from build123d import *

# Parameters (mm, degrees)
CYLINDER031_R              = 3.1
CYLINDER031_DEPTH          = 32.5
EXTRUDE002_DEPTH           = 10
CYLINDER038_R              = 2.5
CYLINDER038_DEPTH          = 23
CYLINDER032_R              = 4
CYLINDER032_DEPTH          = 10
EXTRUDE005_DEPTH           = 4
EXTRUDE005_PLACEMENT_ANGLE = 90
CYLINDER019_R              = 11.1
CYLINDER019_DEPTH          = 10
CYLINDER015_R              = 1.6
CYLINDER015_DEPTH          = 10
CYLINDER016_R              = 1.6
CYLINDER016_DEPTH          = 10
CYLINDER017_R              = 1.6
CYLINDER017_DEPTH          = 10
CYLINDER018_R              = 1.6
CYLINDER018_DEPTH          = 10
BOX002_W                   = 44
BOX002_H                   = 4
BOX002_DEPTH               = 43
EXTRUDE001_DEPTH           = 4
EXTRUDE006_DEPTH           = 5.9
EXTRUDE006_PLACEMENT_ANGLE = 90
CYLINDER021_R              = 6
CYLINDER021_DEPTH          = 6
CYLINDER020_R              = 2.1
CYLINDER020_DEPTH          = 10
BOX003_W                   = 66
BOX003_H                   = 25
BOX003_DEPTH               = 4
BOX_W                      = 19
BOX_H                      = 25
BOX_DEPTH                  = 4
CYLINDER028_R              = 11.1
CYLINDER028_DEPTH          = 10
CYLINDER025_R              = 1.6
CYLINDER025_DEPTH          = 10
CYLINDER024_R              = 1.6
CYLINDER024_DEPTH          = 10
CYLINDER023_R              = 1.6
CYLINDER023_DEPTH          = 10
CYLINDER029_R              = 1.6
CYLINDER029_DEPTH          = 10
BOX005_W                   = 44
BOX005_H                   = 4
BOX005_DEPTH               = 43


with BuildPart() as cylinder031:
    # Cylinder031 → Cylinder031 (new body)
    with BuildSketch(Plane(origin=(7.1, -2.84478, 23.5), x_dir=(1, 0, 0), z_dir=(0, 1, 0))):
        Circle(CYLINDER031_R)
    extrude(amount=CYLINDER031_DEPTH)


with BuildPart() as extrude002:
    # Sketch001 → Extrude002 (new body)
    with BuildSketch(Plane.XY):
        with BuildLine():
            ThreePointArc((35.736492, 10), (36.2, 15), (35.736492, 20))
            ThreePointArc((35.736492, 20), (33.490746, 22.111711), (31.244999, 20))
            ThreePointArc((31.244999, 10), (31.8, 15), (31.244999, 20))
            ThreePointArc((31.244999, 10), (33.490746, 7.888289), (35.736492, 10))
        make_face()
    extrude(amount=-EXTRUDE002_DEPTH)


with BuildPart() as extrude002_1:
    # Extrude002 placement: moved
    add(extrude002.part.moved(Location((0, 0, 8))))


with BuildPart() as cylinder038:
    # Cylinder038 → Cylinder038 (new body)
    with BuildSketch(Plane(origin=(6, 27, 39), x_dir=(1, 0, 0), z_dir=(0, -1, 0))):
        Circle(CYLINDER038_R)
    extrude(amount=CYLINDER038_DEPTH)


with BuildPart() as cylinder032:
    # Cylinder032 → Cylinder032 (new body)
    with BuildSketch(Plane(origin=(6, 27, 8), x_dir=(1, 0, 0), z_dir=(0, -1, 0))):
        Circle(CYLINDER032_R)
    extrude(amount=CYLINDER032_DEPTH)


with BuildPart() as extrude005:
    # Sketch003 → Extrude005 (new body)
    with BuildSketch(Plane.YZ):
        Polygon((0, 0), (0, 43), (4, 43), (25, 4), (25, 0), align=None)
    extrude(amount=EXTRUDE005_DEPTH)


with BuildPart() as extrude005_1:
    # Extrude005 placement: moved
    add(extrude005.part.moved(Location((4, 0, 0))).rotate(Axis((4, 0, 0), (0, 0, 1)), EXTRUDE005_PLACEMENT_ANGLE))


with BuildPart() as cylinder019:
    # Cylinder019 → Cylinder019 (new body)
    with BuildSketch(Plane(origin=(21.5, -2, 23.5), x_dir=(1, 0, 0), z_dir=(0, 1, 0))):
        Circle(CYLINDER019_R)
    extrude(amount=CYLINDER019_DEPTH)


with BuildPart() as cylinder015:
    # Cylinder015 → Cylinder015 (new body)
    with BuildSketch(Plane(origin=(37, -3, 8), x_dir=(1, 0, 0), z_dir=(0, 1, 0))):
        Circle(CYLINDER015_R)
    extrude(amount=CYLINDER015_DEPTH)


with BuildPart() as cylinder016:
    # Cylinder016 → Cylinder016 (new body)
    with BuildSketch(Plane(origin=(6, -3, 8), x_dir=(1, 0, 0), z_dir=(0, 1, 0))):
        Circle(CYLINDER016_R)
    extrude(amount=CYLINDER016_DEPTH)


with BuildPart() as cylinder017:
    # Cylinder017 → Cylinder017 (new body)
    with BuildSketch(Plane(origin=(6, -3, 39), x_dir=(1, 0, 0), z_dir=(0, 1, 0))):
        Circle(CYLINDER017_R)
    extrude(amount=CYLINDER017_DEPTH)


with BuildPart() as cylinder018:
    # Cylinder018 → Cylinder018 (new body)
    with BuildSketch(Plane(origin=(37, -3, 39), x_dir=(1, 0, 0), z_dir=(0, 1, 0))):
        Circle(CYLINDER018_R)
    extrude(amount=CYLINDER018_DEPTH)


with BuildPart() as cut014:
    # Box002 → Box002 (new body)
    with BuildSketch(Plane.XY):
        with Locations((22, 2)):
            Rectangle(BOX002_W, BOX002_H)
    extrude(amount=BOX002_DEPTH)

    # Cut010: cut Cylinder018
    add(cylinder018.part, mode=Mode.SUBTRACT)

    # Cut011: cut Cylinder017
    add(cylinder017.part, mode=Mode.SUBTRACT)

    # Cut012: cut Cylinder016
    add(cylinder016.part, mode=Mode.SUBTRACT)

    # Cut013: cut Cylinder015
    add(cylinder015.part, mode=Mode.SUBTRACT)

    # Cut014: cut Cylinder019
    add(cylinder019.part, mode=Mode.SUBTRACT)


with BuildPart() as extrude001:
    # Sketch → Extrude001 (new body)
    with BuildSketch(Plane.YZ):
        Polygon((0, 0), (0, 43), (4, 43), (25, 4), (25, 0), align=None)
    extrude(amount=EXTRUDE001_DEPTH)


with BuildPart() as extrude001_1:
    # Extrude001 placement: moved
    add(extrude001.part.moved(Location((41, 0, 0))))


with BuildPart() as extrude006:
    # Sketch004 → Extrude006 (new body)
    with BuildSketch(Plane.YZ):
        Polygon((0, 0), (0, 43), (19, 43), (40, 4), (40, 0), align=None)
    extrude(amount=EXTRUDE006_DEPTH)


with BuildPart() as extrude006_1:
    # Extrude006 placement: moved
    add(extrude006.part.moved(Location((19.2, 19.1, 0))).rotate(Axis((19.2, 19.1, 0), (0, 0, 1)), EXTRUDE006_PLACEMENT_ANGLE))


with BuildPart() as cylinder021:
    # Cylinder021 → Cylinder021 (new body)
    with BuildSketch(Plane.XY.offset(10)):
        Circle(CYLINDER021_R)
    extrude(amount=CYLINDER021_DEPTH)


with BuildPart() as fusion004:
    # Cylinder020 → Cylinder020 (new body)
    with BuildSketch(Plane.XY):
        Circle(CYLINDER020_R)
    extrude(amount=CYLINDER020_DEPTH)

    # Fusion004: union Cylinder021
    add(cylinder021.part)


with BuildPart() as fusion004_1:
    # Fusion004 placement: moved
    add(fusion004.part.moved(Location((-7, 12, -7))))


with BuildPart() as cut029:
    # Box003 → Box003 (new body)
    with BuildSketch(Plane(origin=(-21, 0, 0), x_dir=(1, 0, 0), z_dir=(0, 0, 1))):
        with Locations((33, 12.5)):
            Rectangle(BOX003_W, BOX003_H)
    extrude(amount=BOX003_DEPTH)

    # Cut: cut Fusion004
    add(fusion004_1.part, mode=Mode.SUBTRACT)

    # Fusion: union Extrude005, Cut014, Extrude001, Extrude006
    add(extrude005_1.part)
    add(cut014.part)
    add(extrude001_1.part)
    add(extrude006_1.part)

    # Cut029: cut Cylinder032
    add(cylinder032.part, mode=Mode.SUBTRACT)


with BuildPart() as box:
    # Box → Box (new body)
    with BuildSketch(Plane(origin=(0.2, 0, 39), x_dir=(1, 0, 0), z_dir=(0, 0, 1))):
        with Locations((9.5, 12.5)):
            Rectangle(BOX_W, BOX_H)
    extrude(amount=BOX_DEPTH)


with BuildPart() as cylinder028:
    # Cylinder028 → Cylinder028 (new body)
    with BuildSketch(Plane(origin=(21.5, -2, 23.5), x_dir=(1, 0, 0), z_dir=(0, 1, 0))):
        Circle(CYLINDER028_R)
    extrude(amount=CYLINDER028_DEPTH)


with BuildPart() as cylinder025:
    # Cylinder025 → Cylinder025 (new body)
    with BuildSketch(Plane(origin=(37, -3, 8), x_dir=(1, 0, 0), z_dir=(0, 1, 0))):
        Circle(CYLINDER025_R)
    extrude(amount=CYLINDER025_DEPTH)


with BuildPart() as cylinder024:
    # Cylinder024 → Cylinder024 (new body)
    with BuildSketch(Plane(origin=(6, -3, 8), x_dir=(1, 0, 0), z_dir=(0, 1, 0))):
        Circle(CYLINDER024_R)
    extrude(amount=CYLINDER024_DEPTH)


with BuildPart() as cylinder023:
    # Cylinder023 → Cylinder023 (new body)
    with BuildSketch(Plane(origin=(6, -3, 39), x_dir=(1, 0, 0), z_dir=(0, 1, 0))):
        Circle(CYLINDER023_R)
    extrude(amount=CYLINDER023_DEPTH)


with BuildPart() as cylinder029:
    # Cylinder029 → Cylinder029 (new body)
    with BuildSketch(Plane(origin=(37, -3, 39), x_dir=(1, 0, 0), z_dir=(0, 1, 0))):
        Circle(CYLINDER029_R)
    extrude(amount=CYLINDER029_DEPTH)


with BuildPart() as cut032:
    # Box005 → Box005 (new body)
    with BuildSketch(Plane.XY):
        with Locations((22, 2)):
            Rectangle(BOX005_W, BOX005_H)
    extrude(amount=BOX005_DEPTH)

    # Cut017: cut Cylinder029
    add(cylinder029.part, mode=Mode.SUBTRACT)

    # Cut018: cut Cylinder023
    add(cylinder023.part, mode=Mode.SUBTRACT)

    # Cut021: cut Cylinder024
    add(cylinder024.part, mode=Mode.SUBTRACT)

    # Cut022: cut Cylinder025
    add(cylinder025.part, mode=Mode.SUBTRACT)

    # Cut016: cut Cylinder028
    add(cylinder028.part, mode=Mode.SUBTRACT)

    # Fusion008: union Box
    add(box.part)

    # Fusion009: union Cut029
    add(cut029.part)

    # Cut030: cut Cylinder038
    add(cylinder038.part, mode=Mode.SUBTRACT)

    # Cut031: cut Extrude002
    add(extrude002_1.part, mode=Mode.SUBTRACT)

    # Cut032: cut Cylinder031
    add(cylinder031.part, mode=Mode.SUBTRACT)


solid = cut032.part
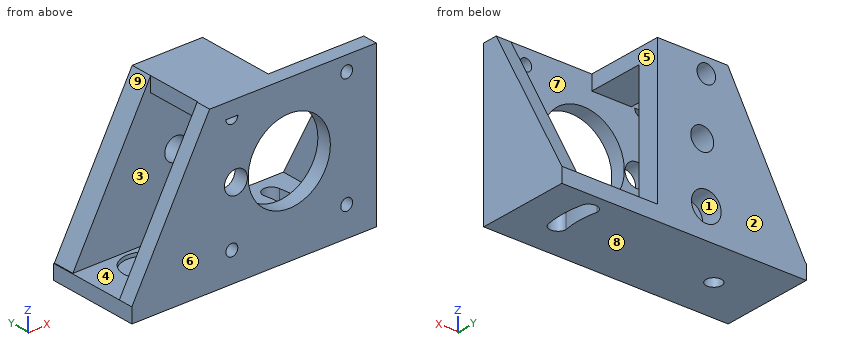
The listing builds one solid part. Answer for the finished solid, in the listing's coordinates (mm). Face numbers are marked on the shaded views. A direction names the side the tool comes from. Coordinates: 2 decimals unless noted, no trailing zeros. Loops run counter-clockwise (first coordinate to the right, second up) from the corner with the lowest first, then second, coordinate; pieces in that order, holes last.
1) Determine the mould class of the marked faces 6, 7, 8 and 9 for opening direction Z: pulls with the +Z half, pulls with the -Z half, needs draft (parallel to the pull), parting line crosses it, or undercut.
2) Flat-ended cylindrical pins translate along their axes: pin 1 Ø5.5 at (x, z) = (7.1, 23.5) entering from -Y (3 decimals); pin 2 Ø4 at (y, z) = (10.5, 38.5) entering from -X; pin 3 Ø3 at (x, y) = (-8.5, 17.5) entering from +Z; pin 4 Ø3 at (x, z) = (34, 23.5) entering from +Y. Find the tip coordinate at first contact, or state that the pin passes through.
3) Find section B-B on x = 21.5. Write down the section's boundary in (y, z), then the cut area to 3 significant figures.
4) A tool of negligible diameter and unlimited length cuts with its end or side. For the marked faces 1, 2, 3, 4 and 5, from which of +Z, -Z, +X, -X, +Y, -Y can it reach the whole face along a straight path? Write none if from no direction.
5) Find section C-C on y = 13.25. Write down the section's boundary in (x, z), then the cut area to 3 significant figures.
6) Find section D-D on z = 11. Write down the section's boundary in (x, y), then the cut area to 3 significant figures.
7) Find the intervals of material crossed by L1, parallel to Z at x = 37, y = 2.6; L2, parallel to Z at x = 1, y = 10.75; L3, parallel to Y at x = -4, z = 11, in increasing order.
8) Find section A-A on z = 23.5. Write down the section's boundary in (x, y), then the cut area to 3 significant figures.
Values:
1. face 6: needs draft
1. face 7: undercut
1. face 8: pulls with the -Z half
1. face 9: pulls with the +Z half
2. pin 1: passes through
2. pin 2: stops at x = 0.2
2. pin 3: stops at z = 4
2. pin 4: stops at y = 4
3. outline: (0, 0) - (25, 0) - (25, 4) - (4, 4) - (4, 12.4) - (0, 12.4) - close; (0, 34.6) - (4, 34.6) - (4, 43) - (0, 43) - close
3. area: 167 mm2
4. face 1: +Y
4. face 2: +Z, -Z, +X, -X, +Y
4. face 3: -X
4. face 4: none
4. face 5: +Z, +Y
5. outline: (-21, 0) - (-8.69, 0) - (-8.69, 3) - (-12.87, 3) - (-12.87, 4) - (-21, 4) - close; (-5.31, 0) - (31.73, 0) - (31.73, 4) - (-1.13, 4) - (-1.13, 3) - (-5.31, 3) - close; (0.2, 39) - (3.5, 39) arc R2.5 cw to (8.5, 39) - (19.2, 39) - (19.2, 43) - (0.2, 43) - close; (36.14, 0) - (45, 0) - (45, 25.82) - (41, 25.82) - (41, 4) - (36.14, 4) - close
5. area: 378 mm2
6. outline: (-17.23, 0) - (45, 0) - (45, 21.23) - (41, 21.23) - (41, 4) - (-17.23, 4) - close; (-17.03, 19.1) - (3.35, 19.1) - (3.35, 25) - (-17.03, 25) - close; (8.65, 19.1) - (19.2, 19.1) - (19.2, 25) - (8.65, 25) - close
6. area: 500 mm2
7. L1: z = 0 to 6.4, 9.6 to 37.4, 40.6 to 43
7. L2: z = 0 to 4, 39 to 43
7. L3: y = 0 to 4, 19.1 to 25
8. outline: (-10.5, 0) - (4, 0) - (4, 4) - (-10.5, 4) - close; (-10.3, 19.1) - (4, 19.1) - (4, 25) - (-10.3, 25) - close; (10.2, 0) - (10.4, 0) - (10.4, 4) - (10.2, 4) - close; (10.2, 19.1) - (19.2, 19.1) - (19.2, 25) - (10.2, 25) - close; (32.6, 0) - (45, 0) - (45, 14.5) - (41, 14.5) - (41, 4) - (32.6, 4) - close
8. area: 288 mm2
